from build123d import *

# Parameters (mm, degrees)
SKETCH_1_R          = 15.5
EXTRUDE_2_DEPTH     = 20
SKETCH_2_W          = 5
SKETCH_2_H          = 40
EXTRUDE_3_DEPTH     = 60
SKETCH_3_R          = 7
EXTRUDE_4_DEPTH     = 2
SKETCH_4_R          = 6
EXTRUDE_5_DEPTH     = 2.5
SKETCH_5_R          = 1.5
CUT_EXTRUDE_1_DEPTH = 45.5
FILLET_1_R          = 10


with BuildPart() as part:
    # Эскиз1 → Бобышка-Вытянуть2 (new body)
    with BuildSketch(Plane(origin=(0, 0, 0), x_dir=(1, 0, 0), z_dir=(0, 1, 0))):
        with BuildLine():
            Line((0, 20), (20, 20))
            Line((20, 20), (20, -20))
            Line((20, -20), (0, -20))
            ThreePointArc((0, -20), (-20, 0), (0, 20))
        make_face()
        Circle(SKETCH_1_R, mode=Mode.SUBTRACT)
    extrude(amount=EXTRUDE_2_DEPTH)

    # Эскиз2 → Бобышка-Вытянуть3 (add)
    with BuildSketch(Plane(origin=(0, 20, 0), x_dir=(1, 0, 0), z_dir=(0, 1, 0))):
        with Locations((17.5, 0)):
            Rectangle(SKETCH_2_W, SKETCH_2_H)
    extrude(amount=EXTRUDE_3_DEPTH)

    # Эскиз3 → Бобышка-Вытянуть4 (add)
    with BuildSketch(Plane(origin=(20, 0, 0), x_dir=(0, 0, -1), z_dir=(1, 0, 0))):
        with Locations((0, 65)):
            Circle(SKETCH_3_R)
    extrude(amount=EXTRUDE_4_DEPTH)

    # Эскиз4 → Бобышка-Вытянуть5 (add)
    with BuildSketch(Plane(origin=(22, 0, 0), x_dir=(0, 0, -1), z_dir=(1, 0, 0))):
        with Locations((0, 65)):
            Circle(SKETCH_4_R)
    extrude(amount=EXTRUDE_5_DEPTH)

    # Эскиз5 → Вырез-Вытянуть1 (cut, through all)
    with BuildSketch(Plane(origin=(24.5, 0, 0), x_dir=(0, 0, -1), z_dir=(1, 0, 0))):
        with Locations((0, 65)):
            Circle(SKETCH_5_R)
    extrude(amount=-CUT_EXTRUDE_1_DEPTH, mode=Mode.SUBTRACT)

    # Скругление1
    fillet_1_edges = [part.edges().sort_by_distance(p)[0] for p in [
        (17.5, 80, -20),
        (17.5, 80, 20),
    ]]
    fillet(fillet_1_edges, radius=FILLET_1_R)


solid = part.part
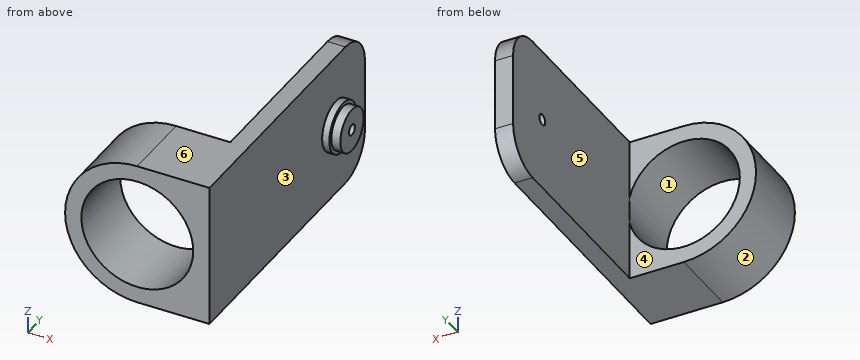
CAD build for the part. Positions are in the model's coordinates, mm. Face numbers are marked on the shaded views. A direction names the side the tool comes from. Coordinates: 2 decimals unless noted, no trailing zeros. Write each loop counter-clockwise with the first axis right and the second up, starting at its lowest first coordinate (ties: lowest second). Pieces come first, ordered by that corner, then holes. Notation, with made-up numbers: M -26,28.25 L 32,28.25 A17 ccw 32,55.25 Z; hole C 43.5,-23 d2. An arc over 180 degrees is marked long. Return JSON: item names as keys, results as strings.
Item 1: Probe line 1 (Y direction, x = 21, z = 0); line 2 (X direction, y = 4, z = 0); line 3 (Z direction, x = -5, y = 18.5). List the from-to ranges inside material, lowest first. Write a range as from..to.
Findings below:
{"line 1": "y = 58..63.5, 66.5..72", "line 2": "x = -20..-15.5, 15.5..20", "line 3": "z = -19.36..-14.67, 14.67..19.36"}
Item 2: Two-plate mould, pull along X, no slides. Class the marked faces 1, 2, 3 and 4: +X half, -X half, draft (parallel to the pull), parting line (faces both ways), or undercut.
Findings below:
{"face 1": "undercut", "face 2": "-X half", "face 3": "+X half", "face 4": "draft"}
Item 3: Slice it at C-C, the plane x = 9.5. Write the cut outline in (y, z), and give its area (3 significant figures).
Findings below:
{"outline": "M 0,-20 L 20,-20 L 20,-12.25 L 0,-12.25 Z; M 0,12.25 L 20,12.25 L 20,20 L 0,20 Z", "area": "310 mm2"}
Item 4: Which spindle directions (+Z, -Z, +X, -X, +Y, -Y) get a long thin tool onto all of the face, cutting with end or side? Do the marked faces 5 and 6. Say none if no direction does.
Findings below:
{"face 5": "+Z, -Z, -X, +Y", "face 6": "+Z, +X, -X, +Y, -Y"}
Item 5: Slice it at D-D, the plane z = -12.5. Write the cut outline in (x, y).
Findings below:
{"outline": "M -15.61,0 L -9.17,0 L -9.17,20 L -15.61,20 Z; M 9.17,0 L 20,0 L 20,79.68 L 15,79.68 L 15,20 L 9.17,20 Z"}
Item 6: Slice it at A-A, the plane z = 0. Write the cut outline in (x, y).
Findings below:
{"outline": "M -20,0 L -15.5,0 L -15.5,20 L -20,20 Z; M 15,20 L 15.5,20 L 15.5,0 L 20,0 L 20,58 L 22,58 L 22,59 L 24.5,59 L 24.5,63.5 L 15,63.5 Z; M 15,66.5 L 24.5,66.5 L 24.5,71 L 22,71 L 22,72 L 20,72 L 20,80 L 15,80 Z"}
Item 7: Drop flat-ended pins along their axis: pin 1 Ø17.5 at (x, z) = (-3, 7) entering from +Y; pin 2 Ø3 at (y, z) = (31.5, 13) entering from -X; pin 3 Ø0.6 at (x, z) = (15, 1.5) entering from -Y. Give the stop position or say it passes through.
Findings below:
{"pin 1": "stops at y = 20", "pin 2": "stops at x = 15", "pin 3": "stops at y = 20"}
Item 8: Slice it at B-B, the plane y = 65. Write the cut outline in (x, z), and give its area (4 significant figures).
Findings below:
{"outline": "M 15,-20 L 20,-20 L 20,-7 L 22,-7 L 22,-6 L 24.5,-6 L 24.5,-1.5 L 15,-1.5 Z; M 15,1.5 L 24.5,1.5 L 24.5,6 L 22,6 L 22,7 L 20,7 L 20,20 L 15,20 Z", "area": "229.5 mm2"}
